Check sheet for the modelled part. Datum: model origin and axes. Units: mm. A direction names the side the tool comes from. Round coordinates to 2 decimals unless told otherwise and drop trailing zeros. Order: outer loops, then holes, each group sorted by start corner. A loop starts at its lowest first (then second) coordinate and runs counter-clockwise, first axis right, second up. Notation, with made-up numbers: (37.5, -12.75) -> (90.5, -12.75) arc R22 ccw to (90.5, 5.25) -> close; hole circle Ø3 at (-26, 69.5). An arc over 180 degrees is marked (long way). Answer as CSV lines item,"result". Start each with the question number.
from build123d import *

# Parameters (mm, degrees)
SKETCH1_W           = 41
SKETCH1_H           = 41
SKETCH1_R           = 1.75
SKETCH1_R_2         = 1.25
BOSS_EXTRUDE1_DEPTH = 2
SKETCH2_W           = 10
SKETCH2_H           = 10
SKETCH2_R           = 1.75
BOSS_EXTRUDE2_DEPTH = 30
FILLET1_R           = 5
SKETCH3_R           = 10.5
CUT_EXTRUDE1_DEPTH  = 1
SKETCH4_R           = 11.5
CUT_EXTRUDE2_DEPTH  = 0.5
BOSS_EXTRUDE3_START = 5
SKETCH6_R           = 12.5
BOSS_EXTRUDE3_DEPTH = 5


with BuildPart() as part:
    # Sketch1 → Boss-Extrude1 (new body)
    with BuildSketch(Plane.XY):
        with Locations((-34.508333333, 4.35625)):
            Rectangle(SKETCH1_W, SKETCH1_H)
        with Locations((-50.008333333, 19.85625)):
            Circle(SKETCH1_R, mode=Mode.SUBTRACT)
        with Locations((-50.008333333, -11.14375)):
            Circle(SKETCH1_R, mode=Mode.SUBTRACT)
        with Locations((-19.008333333, -11.14375)):
            Circle(SKETCH1_R, mode=Mode.SUBTRACT)
        with Locations((-19.008333333, 19.85625)):
            Circle(SKETCH1_R, mode=Mode.SUBTRACT)
        with Locations((-34.508333333, 4.35625)):
            Circle(SKETCH1_R_2, mode=Mode.SUBTRACT)
    extrude(amount=BOSS_EXTRUDE1_DEPTH)

    # Sketch2 → Boss-Extrude2 (add)
    # profile 1 of 4: a face of its own
    with BuildSketch(Plane.XY.offset(2)):
        with Locations((-50.008333333, 19.85625)):
            Rectangle(SKETCH2_W, SKETCH2_H)
        with Locations((-50.008333333, 19.85625)):
            Circle(SKETCH2_R, mode=Mode.SUBTRACT)
    # profile 2 of 4: a face of its own
    with BuildSketch(Plane.XY.offset(2)):
        with Locations((-50.008333333, -11.14375)):
            Rectangle(SKETCH2_W, SKETCH2_H)
        with Locations((-50.008333333, -11.14375)):
            Circle(SKETCH2_R, mode=Mode.SUBTRACT)
    # profile 3 of 4: a face of its own
    with BuildSketch(Plane.XY.offset(2)):
        with Locations((-19.008333333, -11.14375)):
            Rectangle(SKETCH2_W, SKETCH2_H)
        with Locations((-19.008333333, -11.14375)):
            Circle(SKETCH2_R, mode=Mode.SUBTRACT)
    # profile 4 of 4: a face of its own
    with BuildSketch(Plane.XY.offset(2)):
        with Locations((-19.008333333, 19.85625)):
            Rectangle(SKETCH2_W, SKETCH2_H)
        with Locations((-19.008333333, 19.85625)):
            Circle(SKETCH2_R, mode=Mode.SUBTRACT)
    extrude(amount=BOSS_EXTRUDE2_DEPTH)

    # Fillet1
    fillet1_edges = [part.edges().sort_by_distance(p)[0] for p in [
        (-24.008333333, 24.85625, 17),
        (-24.008333333, -6.14375, 17),
        (-55.008333333, -6.14375, 17),
        (-55.008333333, 14.85625, 17),
        (-45.008333333, 24.85625, 17),
        (-45.008333333, -6.14375, 17),
        (-45.008333333, -16.14375, 17),
        (-24.008333333, -16.14375, 17),
        (-14.008333333, -6.14375, 17),
        (-14.008333333, 14.85625, 17),
        (-24.008333333, 14.85625, 17),
        (-45.008333333, 14.85625, 17),
        (-14.008333333, -16.14375, 16),
        (-14.008333333, 24.85625, 16),
        (-55.008333333, -16.14375, 16),
        (-55.008333333, 24.85625, 16),
    ]]
    fillet(fillet1_edges, radius=FILLET1_R - 0.0001)  # a hair under: the kernel refuses the full size

    # Sketch3 → Cut-Extrude1 (cut)
    with BuildSketch(Plane.XY.offset(2)):
        with Locations((-34.508333333, 4.35625)):
            Circle(SKETCH3_R)
    extrude(amount=-CUT_EXTRUDE1_DEPTH, mode=Mode.SUBTRACT)

    # Sketch4 → Cut-Extrude2 (cut)
    with BuildSketch(Plane.XY.offset(2)):
        with Locations((-34.508333333, 4.35625)):
            Circle(SKETCH4_R)
    extrude(amount=-CUT_EXTRUDE2_DEPTH, mode=Mode.SUBTRACT)

    # Sketch6 → Boss-Extrude3 (add)
    with BuildSketch(Plane.XY.offset(2).offset(BOSS_EXTRUDE3_START)):
        with Locations((-34.508333333, 4.35625)):
            Circle(SKETCH6_R)
        with BuildLine():
            ThreePointArc((-23.008333333, 4.35625), (-32.058371909, -6.879749689), (-44.964453163, -0.431187531))
            ThreePointArc((-44.964453163, -0.431187531), (-36.958294758, 15.592249689), (-23.008333333, 4.35625))
        make_face(mode=Mode.SUBTRACT)
    extrude(amount=-BOSS_EXTRUDE3_DEPTH)


solid = part.part
1) Section check B-B on y = -14. Record the cut outline in (x, z).
2) Section check A-A on x = -51. Record the cut outline in (y, z), then the cut area to 3 significant figures.
3) Access from +Z, -Z, +X, -X, +Y, -Y to the whole of each face (thin tool, end or side, straight path). Record for faces 1 (the face through (-17.39, -11.81, 15.78)), 2 (the face through (-17, -11, 32)), 3 (the face through (-53.583, -7.647, 17.21)), 4 (the face through (-15.434, 16.36, 17.21)), 5 (the face through (-42.841, -2.033, 1.254)).
4) Section check D-D on x = -40.5. Record the cut outline in (y, z), then the cut area to 3 significant figures.
5) Depth check by flat-ended pin: pin 1 Ø8 at (x, y) = (-36, 2) entering from -Z; pin 2 Ø4 at (x, z) = (-28, 7.5) entering from +Y; pin 3 Ø10.5 at (x, y) = (-38, 1.5) entering from +Z; pin 4 Ø18.5 at (x, y) = (-37, 1) entering from +Z. Enter the tip coordinate at first touch or a pass-through.
6) Mould release check, pull along X, two halves, no side actions. Record for faces 6 (the face through (-44, 14, 2)), 7 (the face through (-53.583, 23.353, 15.776)), 8 (the face through (-35, 24.856, 1)): released by +X, released by -X, zero draft, split by the parting line, or undercut.
7) Material ranges on line 1 along X through (y, z) = (-11, 1.5); line 2 along X through (y, z) = (-12, 26); line 3 along Y through (x, z) = (-18.5, 22), recorded low to high.
8) Section check C-C on z = 28.5. Count the separate pieces of the cut face and the enclosed holes in it, then the cut area to 3 significant figures.
Solutions:
1,outline,"(-54.11, 0) -> (-14.9, 0) -> (-14.9, 32) -> (-23.11, 32) -> (-23.11, 2) -> (-45.9, 2) -> (-45.9, 32) -> (-54.11, 32) -> close"
2,outline,"(-16.04, 0) -> (-12.59, 0) -> (-12.59, 32) -> (-16.04, 32) -> close; (-9.7, 0) -> (18.41, 0) -> (18.41, 32) -> (14.96, 32) -> (14.96, 2) -> (-6.24, 2) -> (-6.24, 32) -> (-9.7, 32) -> close; (21.3, 0) -> (24.76, 0) -> (24.76, 32) -> (21.3, 32) -> close"
2,area,"485 mm^2"
3,face 1,"+Z, -Z"
3,face 2,"+Z, +X, -X, +Y, -Y"
3,face 3,"+Z, -X"
3,face 4,"+Z, +X"
3,face 5,"+Z"
4,outline,"(-16.14, 0) -> (24.86, 0) -> (24.86, 2) -> (15.33, 2) -> (15.33, 7) -> (14.17, 7) -> (14.17, 1.5) -> (12.98, 1.5) -> (12.98, 1) -> (-4.27, 1) -> (-4.27, 1.5) -> (-5.46, 1.5) -> (-5.46, 7) -> (-6.61, 7) -> (-6.61, 2) -> (-16.14, 2) -> close"
4,area,"75.1 mm^2"
5,pin 1,"stops at z = 0"
5,pin 2,"stops at y = 15.99"
5,pin 3,"stops at z = 1"
5,pin 4,"stops at z = 7"
6,face 6,"undercut"
6,face 7,"released by -X"
6,face 8,"zero draft"
7,line 1,"x = -55.01 to -51.75, -48.26 to -20.75, -17.26 to -14.01"
7,line 2,"x = -54.93 to -51.53, -48.48 to -45.08, -23.93 to -20.53, -17.48 to -14.08"
7,line 3,"y = -16.12 to -12.82, -9.47 to -6.17, 14.88 to 18.18, 21.53 to 24.83"
8,separate pieces,"4"
8,enclosed holes,"4"
8,area,"276 mm^2"
